Source: three-view drawing plus pictorial views. Frame: mm from the lowest corner of the part. Give positions to 0.01 mm unless a question says otherwise; leave off trailing zeros. Loops run counter-clockwise (first coordinate to the right, second up) from the corner with the lowest first, then second, coordinate; pieces in that order, holes last. Notation, with made-up numbers: (40, -0.5) - (80, -0.5) arc R28 ccw to (80, 25.5) - close; hole circle Ø4 at (72, 45). An arc over 180 degrees is marked (long way). Put each result on its own line as item: value.
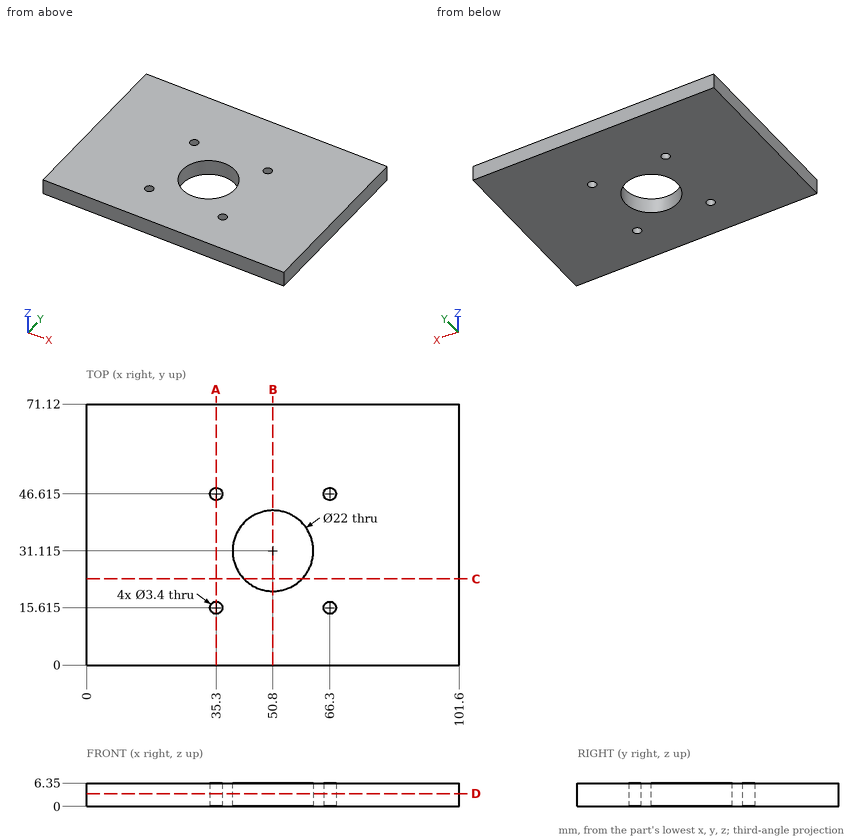
1) Section query B-B, the plane x = 50.8. Output: boundary loops of the cut face in (y, z) (3 decimals), plus the area to 3 significant figures.
Check result:
outline: (0, 0) - (20.115, 0) - (20.115, 6.35) - (0, 6.35) - close; (42.115, 0) - (71.12, 0) - (71.12, 6.35) - (42.115, 6.35) - close
area: 312 mm²
2) Section query C-C, the plane y = 23.5. Output: boundary loops of the cut face in (x, z).
Check result:
outline: (0, 0) - (42.86, 0) - (42.86, 6.35) - (0, 6.35) - close; (58.74, 0) - (101.6, 0) - (101.6, 6.35) - (58.74, 6.35) - close
3) Section query A-A, the plane x = 35.3. Output: boundary loops of the cut face in (y, z) (3 decimals), plus the area to 3 significant figures.
Check result:
outline: (0, 0) - (13.915, 0) - (13.915, 6.35) - (0, 6.35) - close; (17.315, 0) - (44.915, 0) - (44.915, 6.35) - (17.315, 6.35) - close; (48.315, 0) - (71.12, 0) - (71.12, 6.35) - (48.315, 6.35) - close
area: 408 mm²
4) Material intervals for line 1 along Y through (x, z) = (35.3, 5) (3 decimals); line 2 along Y through (x, z) = (34.5, 3.25) (3 decimals); line 3 along X through (y, z) = (30.5, 0.5), sorted ascending. Write a range as [from, to].
Check result:
line 1: [0, 13.915], [17.315, 44.915], [48.315, 71.12]
line 2: [0, 14.115], [17.115, 45.115], [48.115, 71.12]
line 3: [0, 39.82], [61.78, 101.6]
5) Section query D-D, the plane z = 3.5. Output: boundary loops of the cut face in (x, y) (3 decimals).
Check result:
outline: (0, 0) - (101.6, 0) - (101.6, 71.12) - (0, 71.12) - close; hole circle Ø3.4 at (35.3, 15.615); hole circle Ø3.4 at (35.3, 46.615); hole circle Ø22 at (50.8, 31.115); hole circle Ø3.4 at (66.3, 15.615); hole circle Ø3.4 at (66.3, 46.615)
